Can you work these out from the model? Positions are in its coordinate system, mm. Face numbers are marked on the shaded views. A direction names the side the tool comes from. Give positions to 0.01 mm unless a question says otherwise; leave off trailing zeros. Order: outer loops, then holes, each group sorted by start corner. A loop starts at its lowest first (then second) coordinate and runs counter-clockwise, first axis right, second up. Notation, with made-up numbers: M -12,11.5 L 23,11.5 A9 cw 23,22.5 Z; hole C -34.5,-32 d6. An arc over 180 degrees is marked long. Use one line per item in the form item = value. Start each with the question number.
1. I want a section at A-A, the plane z = 212. List the corners of the cut face in (x, y) for me, and give its area (3 significant figures).
2. For the marked faces 1 and 2, which set-ups out of +Z, -Z, +X, -X, +Y, -Y let a thin tool reach every point of the face, with its end or its side?
3. I want a section at B-B, the plane x = -107. List the corners of the cut face in (y, z) for me.
4. We'd pull the mould along X, two halves only. Please class the marked faces 3, 4, 5 and 6: +X half, -X half, draft (parallel to the pull), parting line (faces both ways), or undercut.
5. Will these pins go through, and if not, where does the flat tip stop? P1, Ø1.5, axis at x = -44.5, z = 31.5, coming from the +Y side; P2, Ø0.5, axis at x = 142, z = 1, coming from the +Y side; P3, Ø3.5, axis at y = 0, z = 212, coming from the -X side; P4, Ø6, axis at x = 98.5, y = -16.5, coming from the -Z side.
6. I need wall thicknesses on L1, parallel to X at y = 19, z = 71.5; L2, parallel to Z at x = -142.2, y = 0; L3, parallel to Z at x = 26, y = -3.5. Which ranges of each line are inside material? Lowest first, please.
7. I want a section at C-C, the plane z = 138. List the corners of the cut face in (x, y) for me.
8. I want a section at D-D, the plane y = -11. List the corners of the cut face in (x, z) for me.
```python
from build123d import *

# Parameters (mm, degrees)
F1_DEPTH  = 30
F5_W      = 282
F5_H      = 120
F6_DEPTH  = 3
F7_W      = 43.7729824334
F7_H      = 28.8367732428
F8_DEPTH  = 200
F9_W      = 426.6595542431
F9_H      = 302.5457262993
F10_DEPTH = 178.83968
F12_DEPTH = 3.8062
F13_R     = 5
F14_DEPTH = 5.03518
F16_DEPTH = 250
F17_R     = 3
F17_R_2   = 2
F17_R_3   = 4
F17_R_4   = 5
F17_R_5   = 6
F17_R_6   = 2.5
F18_DEPTH = 160


with BuildPart() as f1:
    # F0 (on Front) → F1 (new body, symmetric)
    with BuildSketch(Plane.XZ):
        Polygon((-143, 230), (-143, 0), (143, 0), (143, 230), (141, 230), (141, 2), (-141, 2), (-141, 230), align=None)
    extrude(amount=F1_DEPTH, both=True)

    # F5 (on line) → F6 (join)
    with BuildSketch(Plane(origin=(0, 9.1354545764, 14.0673664308), x_dir=(1, 0, 0), z_dir=(0, 0.544639035, 0.8386705679))):
        Rectangle(F5_W, F5_H)
    extrude(amount=F6_DEPTH)

    # F7 (on Right) → F8 (cut, symmetric)
    with BuildSketch(Plane.YZ):
        with Locations((51.9040221355, -7.7139467467)):
            Rectangle(F7_W, F7_H)
    extrude(amount=F8_DEPTH, both=True, mode=Mode.SUBTRACT)

    # F9 (on line) → F10 (cut)
    with BuildSketch(Plane(origin=(0, 9.1354545764, 14.0673664308), x_dir=(1, 0, 0), z_dir=(0, 0.544639035, 0.8386705679))):
        Rectangle(F9_W, F9_H)
    extrude(amount=-F10_DEPTH, mode=Mode.SUBTRACT)

    # F11 (on line) → F12 (cut)
    with BuildSketch(Plane(origin=(0, 9.1354545764, 14.0673664308), x_dir=(1, 0, 0), z_dir=(0, 0.544639035, 0.8386705679))):
        with BuildLine():
            Line((-35.8740181322, -48.1499919599), (-147.1929774903, -48.1499919599))
            Line((-147.1929774903, -48.1499919599), (-147.1929774903, -83.3061976281))
            Line((-147.1929774903, -83.3061976281), (146.3554831755, -83.3061976281))
            Line((146.3554831755, -83.3061976281), (146.3554831755, -48.1499919599))
            Line((146.3554831755, -48.1499919599), (35.8740181322, -48.1499919599))
            ThreePointArc((35.8740181322, -48.1499919599), (0, -60.0447075327), (-35.8740181322, -48.1499919599))
        make_face()
    extrude(amount=F12_DEPTH, mode=Mode.SUBTRACT)

    # F13 (on line) → F14 (cut)
    with BuildSketch(Plane(origin=(0, 9.1354545764, 14.0673664308), x_dir=(1, 0, 0), z_dir=(0, 0.544639035, 0.8386705679))):
        with Locations((0, -10.8780780347)):
            Circle(F13_R)
        with BuildLine():
            ThreePointArc((0, -40.4202267205), (2.1637354956, -42.2413960688), (2.9932901548, -44.9451431276))
            ThreePointArc((2.9932901548, -44.9451431276), (4.9922933203, -44.7672054535), (6.9813866372, -44.5004035637))
            ThreePointArc((6.9813866372, -44.5004035637), (5.3606612707, -41.2920368002), (2.0064089085, -40))
            Line((2.0064089085, -40), (1.8917191601, -40))
            ThreePointArc((1.8917191601, -40), (1.8377091807, -40.0025177501), (1.7836958509, -40.0049625733))
            ThreePointArc((1.7836958509, -40.0049625733), (0.8726729327, -40.1302317573), (0, -40.4202267205))
        make_face()
        with BuildLine():
            ThreePointArc((6.9813866372, -44.5004035637), (4.9922933203, -44.7672054535), (2.9932901548, -44.9451431276))
            ThreePointArc((2.9932901548, -44.9451431276), (2.1937501825, -47.7126856822), (0, -49.5797732795))
            ThreePointArc((0, -49.5797732795), (0.9814372986, -49.8938158117), (2.0064089085, -50))
            ThreePointArc((2.0064089085, -50), (2.1177930783, -49.9987592027), (2.2291219661, -49.9950374267))
            ThreePointArc((2.2291219661, -49.9950374267), (5.7881740651, -48.2708182922), (6.9813866372, -44.5004035637))
        make_face()
        with BuildLine():
            ThreePointArc((2.0064089085, -40), (5.3606612707, -41.2920368002), (6.9813866372, -44.5004035637))
            ThreePointArc((6.9813866372, -44.5004035637), (5.7881740651, -48.2708182922), (2.2291219661, -49.9950374267))
            ThreePointArc((2.2291219661, -49.9950374267), (16.8043601395, -47.1390096665), (29.8994669009, -40.1309684792))
            ThreePointArc((29.8994669009, -40.1309684792), (30.9217030257, -33.1341811231), (23.9249156696, -32.1119449984))
            ThreePointArc((23.9249156696, -32.1119449984), (13.4974075811, -37.7014401578), (1.8917191601, -40))
            Line((1.8917191601, -40), (2.0064089085, -40))
        make_face()
        with BuildLine():
            ThreePointArc((-1.7836958509, -40.0049625733), (-0.8726729327, -40.1302317574), (0, -40.4202267205))
            ThreePointArc((0, -40.4202267205), (0.8726729327, -40.1302317573), (1.7836958509, -40.0049625733))
            ThreePointArc((1.7836958509, -40.0049625733), (1.8377091807, -40.0025177501), (1.8917191601, -40))
            Line((1.8917191601, -40), (-1.8917191601, -40))
            ThreePointArc((-1.8917191601, -40), (-1.8377091807, -40.0025177501), (-1.7836958509, -40.0049625733))
        make_face()
        with BuildLine():
            ThreePointArc((-2.9932901548, -44.9451431276), (-2.1637354956, -42.2413960688), (0, -40.4202267205))
            ThreePointArc((0, -40.4202267205), (-0.8726729327, -40.1302317574), (-1.7836958509, -40.0049625733))
            ThreePointArc((-1.7836958509, -40.0049625733), (-1.8377091807, -40.0025177501), (-1.8917191601, -40))
            Line((-1.8917191601, -40), (-2.0064089085, -40))
            ThreePointArc((-2.0064089085, -40), (-5.3606612707, -41.2920368002), (-6.9813866372, -44.5004035637))
            ThreePointArc((-6.9813866372, -44.5004035637), (-4.9922933203, -44.7672054535), (-2.9932901548, -44.9451431276))
        make_face()
        with BuildLine():
            ThreePointArc((-2.0064089085, -50), (-0.9814372986, -49.8938158117), (0, -49.5797732795))
            ThreePointArc((0, -49.5797732795), (-2.1937501825, -47.7126856822), (-2.9932901548, -44.9451431276))
            ThreePointArc((-2.9932901548, -44.9451431276), (-4.9922933203, -44.7672054535), (-6.9813866372, -44.5004035637))
            ThreePointArc((-6.9813866372, -44.5004035637), (-5.7881740651, -48.2708182922), (-2.2291219661, -49.9950374267))
            ThreePointArc((-2.2291219661, -49.9950374267), (-2.1177930783, -49.9987592027), (-2.0064089085, -50))
        make_face()
        with BuildLine():
            ThreePointArc((2.0064089085, -50), (0.9814372986, -49.8938158117), (0, -49.5797732795))
            ThreePointArc((0, -49.5797732795), (-0.9814372986, -49.8938158117), (-2.0064089085, -50))
            Line((-2.0064089085, -50), (2.0064089085, -50))
        make_face()
        with BuildLine():
            ThreePointArc((-2.2291219661, -49.9950374267), (-5.7881740651, -48.2708182922), (-6.9813866372, -44.5004035637))
            ThreePointArc((-6.9813866372, -44.5004035637), (-5.3606612707, -41.2920368002), (-2.0064089085, -40))
            Line((-2.0064089085, -40), (-1.8917191601, -40))
            ThreePointArc((-1.8917191601, -40), (-13.4974075811, -37.7014401578), (-23.9249156696, -32.1119449984))
            ThreePointArc((-23.9249156696, -32.1119449984), (-30.9217030257, -33.1341811231), (-29.8994669009, -40.1309684792))
            ThreePointArc((-29.8994669009, -40.1309684792), (-16.8043601395, -47.1390096665), (-2.2291219661, -49.9950374267))
        make_face()
        with BuildLine():
            ThreePointArc((63, -6.1009786912), (58, -11.1009786912), (63, -16.1009786912))
            Line((63, -16.1009786912), (113, -16.1009786912))
            ThreePointArc((113, -16.1009786912), (118, -11.1009786912), (113, -6.1009786912))
            Line((113, -6.1009786912), (63, -6.1009786912))
        make_face()
        with BuildLine():
            ThreePointArc((-63, -16.1009786912), (-58, -11.1009786912), (-63, -6.1009786912))
            Line((-63, -6.1009786912), (-113, -6.1009786912))
            ThreePointArc((-113, -6.1009786912), (-118, -11.1009786912), (-113, -16.1009786912))
            Line((-113, -16.1009786912), (-63, -16.1009786912))
        make_face()
        with BuildLine():
            Line((-2.0064089085, -45), (2.0064089085, -45))
            ThreePointArc((2.0064089085, -45), (2.5, -44.9752785062), (2.9932901548, -44.9451431276))
            ThreePointArc((2.9932901548, -44.9451431276), (2.1637354956, -42.2413960688), (0, -40.4202267205))
            ThreePointArc((0, -40.4202267205), (-2.1637354956, -42.2413960688), (-2.9932901548, -44.9451431276))
            ThreePointArc((-2.9932901548, -44.9451431276), (-2.5, -44.9752785062), (-2.0064089085, -45))
        make_face()
        with BuildLine():
            ThreePointArc((2.9932901548, -44.9451431276), (2.5, -44.9752785062), (2.0064089085, -45))
            Line((2.0064089085, -45), (-2.0064089085, -45))
            ThreePointArc((-2.0064089085, -45), (-2.5, -44.9752785062), (-2.9932901548, -44.9451431276))
            ThreePointArc((-2.9932901548, -44.9451431276), (-2.1937501825, -47.7126856822), (0, -49.5797732795))
            ThreePointArc((0, -49.5797732795), (2.1937501825, -47.7126856822), (2.9932901548, -44.9451431276))
        make_face()
    extrude(amount=F14_DEPTH, mode=Mode.SUBTRACT)

    # F15 (on Right) → F16 (cut, symmetric)
    with BuildSketch(Plane.YZ):
        with BuildLine():
            ThreePointArc((-16.3768878257, 204.5302245586), (-0.0754798588, 229.9998417435), (16.4389577327, 204.6678332901))
            ThreePointArc((16.4389577327, 204.6678332901), (15.7076024778, 202.2373750115), (15.6116939447, 199.7010766248))
            Line((15.6116939447, 199.7010766248), (30.1540475339, 0))
            Line((30.1540475339, 0), (77.6267153025, 0))
            Line((77.6267153025, 0), (77.6267153025, 43.465353315))
            Line((77.6267153025, 43.465353315), (77.6267153025, 273.465353315))
            Line((77.6267153025, 273.465353315), (-42.3732846975, 273.465353315))
            Line((-42.3732846975, 273.465353315), (-42.3732846975, 52.13252455))
            Line((-42.3732846975, 52.13252455), (-29.599333182, 43.482657522))
            Line((-29.599333182, 43.482657522), (-15.5156644868, 199.4811984753))
            ThreePointArc((-15.5156644868, 199.4811984753), (-15.6175338066, 202.0617858131), (-16.3768878257, 204.5302245586))
        make_face()
    extrude(amount=F16_DEPTH, both=True, mode=Mode.SUBTRACT)

    # F17 (on Right) → F18 (cut, symmetric)
    with BuildSketch(Plane.YZ):
        with Locations((0, 212)):
            Circle(F17_R)
        with Locations((0, 194.167)):
            Circle(F17_R_2)
        with Locations((0, 148.167)):
            Circle(F17_R_3)
        with Locations((0, 102.167)):
            Circle(F17_R_4)
        with Locations((0, 59.167)):
            Circle(F17_R_5)
        with Locations((20, 29.167)):
            Circle(F17_R_6)
    extrude(amount=F18_DEPTH, both=True, mode=Mode.SUBTRACT)


solid = f1.part
```
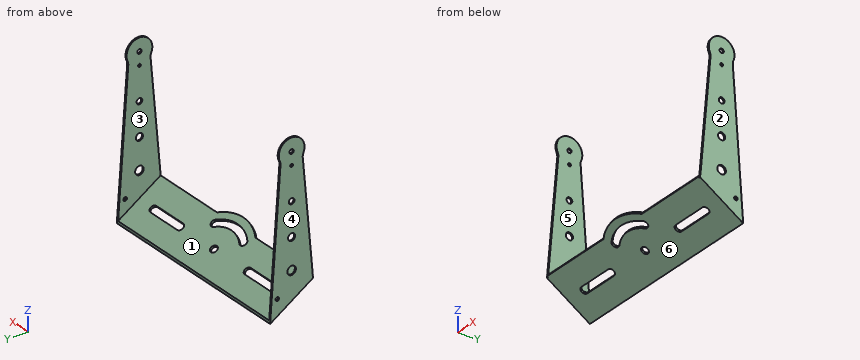
Check result:
q1.outline = M -143,-18 L -141,-18 L -141,-3 L -143,-3 Z; M -143,3 L -141,3 L -141,18 L -143,18 Z; M 141,-18 L 143,-18 L 143,-3 L 141,-3 Z; M 141,3 L 143,3 L 143,18 L 141,18 Z
q1.area = 120 mm2
q2.face_1 = +Z, +Y
q2.face_2 = +Z, -Z, +X, +Y, -Y
q3.outline = M -31.25,40.29 L -4.37,22.84 L -2.73,25.35 L -29.61,42.81 Z; M 4.02,17.39 L 30.02,0.51 L 30.02,1.87 L 29.85,4.19 L 5.65,19.91 Z
q4.face_3 = undercut
q4.face_4 = -X half
q4.face_5 = undercut
q4.face_6 = draft
q5.P1 = -11.05
q5.P2 = 30
q5.P3 = through
q5.P4 = 28.77
q6.L1 = -143 to -141, 141 to 143
q6.L2 = 20 to 53.17, 65.17 to 97.17, 107.17 to 144.17, 152.17 to 192.17, 196.17 to 209, 215 to 230
q6.L3 = 22.27 to 25.85
q7.outline = M -143,-21.07 L -141,-21.07 L -141,20.1 L -143,20.1 Z; M 141,-21.07 L 143,-21.07 L 143,20.1 L 141,20.1 Z
q8.outline = M -143,27.14 L 143,27.14 L 143,226.25 L 141,226.25 L 141,30.72 L -141,30.72 L -141,226.25 L -143,226.25 Z
